Input: part model. Units: mm. Frame: model coordinates. Round coordinates to 2 decimals unless told otherwise and drop trailing zeros. Order: outer loops, then holes, each group sorted by start corner. A loop starts at its lowest first (then second) coordinate and runs counter-clockwise, first axis right, second up. Notation, with made-up numbers: (12, 81) - (16, 81) arc R26 cw to (16, 106) - close; hole circle Ø10 at (-26, -18.75). An arc over 180 degrees is marked (long way). One line per item, written item: value. Start each with the question number.
from build123d import *

# Parameters (mm, degrees)
F0_W     = 50
F0_H     = 50
F1_DEPTH = 30
F4_W     = 50
F4_H     = 50
F5_DEPTH = 10
F6_DEPTH = 10


with BuildPart() as f1:
    # F0 (on Top) → F1 (new body)
    with BuildSketch(Plane.XY):
        with Locations((25, 25)):
            Rectangle(F0_W, F0_H)
    extrude(amount=F1_DEPTH)

    # F2 (on face) → F3 (revolve, cut)
    with BuildSketch(Plane(origin=(0, 0, 0), x_dir=(1, 0, 0), z_dir=(0, 0, -1))):
        with BuildLine():
            ThreePointArc((25, -40), (35.6066017178, -35.6066017178), (40, -25))
            ThreePointArc((40, -25), (35.6066017178, -14.3933982822), (25, -10))
            Line((25, -10), (25, -40))
        make_face()
    revolve(axis=Axis((25, 25, 0), (0, 1, 0)), mode=Mode.SUBTRACT)

    # F4 (on face) → F5 (join)
    with BuildSketch(Plane(origin=(0, 0, 0), x_dir=(1, 0, 0), z_dir=(0, 0, -1))):
        with Locations((25, -25)):
            Rectangle(F4_W, F4_H)
        with BuildLine():
            ThreePointArc((25, -10), (40, -25), (25, -40))
            ThreePointArc((25, -40), (10, -25), (25, -10))
        make_face(mode=Mode.SUBTRACT)
    extrude(amount=F5_DEPTH)

    # F6 (cut): a face of the model
    f6_faces = [f1.faces().sort_by_distance(p)[0] for p in [
        (25, 25, 30),
    ]]
    extrude(f6_faces, amount=-F6_DEPTH, mode=Mode.SUBTRACT)


solid = f1.part
1. Line query: line 1 (X direction, y = 25, z = -5); line 2 (X direction, y = 34, z = 11). Output: solid intervals per line, ascending. Write a range as from..to.
2. Section A-A (z = -2.75). Return the cut outline in (x, y).
3. Section C-C (x = 25). Return the cut outline in (y, z), then the cut area to 3 significant figures.
4. Section B-B (y = 34). Return the cut outline in (x, z), then the cut area to 3 significant figures.
5. Pull-direction query (Y, two-part tool) for faces 1 (the face through (25, 50, 5)), 2 (the face through (39.643, 21.748, -4.93)), 3 (the face through (25, 0, 5)), 4 (the face through (25, 25, 20)); classes: released by +Y, released by -Y, zero draft, split by the parting line, or undercut.
6. Section D-D (z = 9.75). Return the cut outline in (x, y).
Solved:
1. line 1: x = 0..10, 40..50
1. line 2: x = 0..20.2, 29.8..50
2. outline: (0, 0) - (50, 0) - (50, 50) - (0, 50) - close; hole circle Ø30 at (25, 25)
3. outline: (0, -10) - (10, -10) - (10, 0) arc R15 cw to (40, 0) - (40, -10) - (50, -10) - (50, 20) - (0, 20) - close
3. area: 847 mm²
4. outline: (0, -10) - (13, -10) - (13, 0) arc R12 cw to (37, 0) - (37, -10) - (50, -10) - (50, 20) - (0, 20) - close
4. area: 1,030 mm²
5. face 1: released by +Y
5. face 2: undercut
5. face 3: released by -Y
5. face 4: zero draft
6. outline: (0, 0) - (50, 0) - (50, 50) - (0, 50) - close; hole circle Ø22.8 at (25, 25)
